Job drawing, mm, ordinate dimensions from the low corner. One solid piece. Coordinates: 2 decimals unless noted, no trailing zeros. Order: outer loops, then holes, each group sorted by start corner. A loop starts at its lowest first (then second) coordinate and runs counter-clockwise, first axis right, second up. Notation, with made-up numbers: (4.25, -6) - (44.25, -6) arc R12 cw to (44.25, 15) - close; hole circle Ø1 at (56.5, -30.75). An arc over 180 degrees is marked (long way). Return JSON: item names as keys, results as strings.
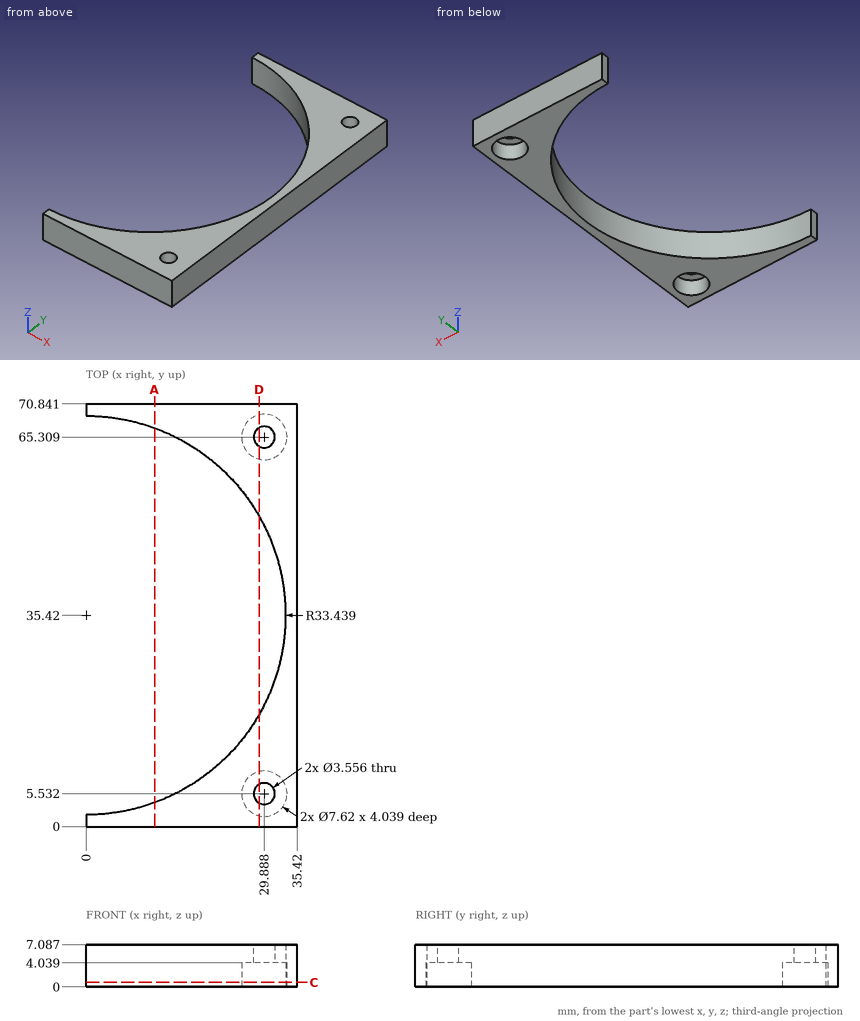
1. Drop flat-ended pins along their axis: pin 1 (7 mm diameter, centred on x = 29.89, y = 65.31, fed in from +Z); pin 2 (2.5 mm diameter, centred on x = 30.5, y = 66, fed in from -Z). Give the stop position or say it passes through.
Check values:
{"pin 1": "z = 7.09", "pin 2": "z = 4.04"}
2. Cut at D-D on x = 29. Give the cut face in (y, z).
Check values:
{"outline": "(0, 0) - (1.83, 0) - (1.83, 4.04) - (3.99, 4.04) - (3.99, 7.09) - (0, 7.09) - close; (7.07, 4.04) - (9.24, 4.04) - (9.24, 0) - (18.77, 0) - (18.77, 7.09) - (7.07, 7.09) - close; (52.07, 0) - (61.6, 0) - (61.6, 4.04) - (63.77, 4.04) - (63.77, 7.09) - (52.07, 7.09) - close; (66.85, 4.04) - (69.01, 4.04) - (69.01, 0) - (70.84, 0) - (70.84, 7.09) - (66.85, 7.09) - close"}
3. Cut at C-C on z = 0.75. Give the cut face in (x, y).
Check values:
{"outline": "(0, 0) - (35.42, 0) - (35.42, 70.84) - (0, 70.84) - (0, 68.86) arc R33.44 cw to (0, 1.98) - close; hole circle Ø7.62 at (29.89, 5.53); hole circle Ø7.62 at (29.89, 65.31)"}
4. Probe L1, parallel to Y at x = 29.5, z = 0.5 (1 decimal); L2, parallel to Y at x = 6, z = 6 (1 decimal); L3, parallel to Y at x = 3, z = 1.5 (1 decimal). List the from-to ranges inside material, lowest first.
Check values:
{"L1": "0 to 1.7, 9.3 to 19.7, 51.2 to 61.5, 69.1 to 70.8", "L2": "0 to 2.5, 68.3 to 70.8", "L3": "0 to 2.1, 68.7 to 70.8"}
5. Cut at A-A on x = 11.5. Give the cut face in (y, z).
Check values:
{"outline": "(0, 0) - (4.02, 0) - (4.02, 7.09) - (0, 7.09) - close; (66.82, 0) - (70.84, 0) - (70.84, 7.09) - (66.82, 7.09) - close"}
